from build123d import *

# Parameters (mm, degrees)
Y_KSEKLIK_EKSTR_ZYON1_DEPTH = 6
KES_EKSTR_ZYON1_DEPTH       = 28.699277969
KES_EKSTR_ZYON1_DEPTH_BACK  = 28.699277969
IZIM2_R                     = 3.5
IZIM3_R                     = 3
KES_EKSTR_ZYON2_DEPTH       = 44


with BuildPart() as part:
    # Çizim1 → Yükseklik-Ekstrüzyon1 (new body)
    with BuildSketch(Plane.XY):
        with BuildLine():
            Line((-16.5, -15), (16.5, -15))
            ThreePointArc((16.5, -15), (20.742640687, -13.242640687), (22.5, -9))
            Line((22.5, -9), (22.5, 9))
            ThreePointArc((22.5, 9), (20.742640687, 13.242640687), (16.5, 15))
            Line((16.5, 15), (-16.5, 15))
            ThreePointArc((-16.5, 15), (-20.742640687, 13.242640687), (-22.5, 9))
            Line((-22.5, 9), (-22.5, -9))
            ThreePointArc((-22.5, -9), (-20.742640687, -13.242640687), (-16.5, -15))
        make_face()
    extrude(amount=Y_KSEKLIK_EKSTR_ZYON1_DEPTH)

    # Çizim2 → Kes-Ekstrüzyon1 (cut, two sides: drawn at the far end of the back side and taken through both)
    with BuildSketch(Plane(origin=(0, 0, 0), x_dir=(0, 0, -1), z_dir=(1, 0, 0)).offset(-KES_EKSTR_ZYON1_DEPTH_BACK)):
        with Locations((-6, 10)):
            Circle(IZIM2_R)
    extrude(amount=KES_EKSTR_ZYON1_DEPTH + KES_EKSTR_ZYON1_DEPTH_BACK, mode=Mode.SUBTRACT)

    # Çizim3 → Kes-Ekstrüzyon2 (cut)
    with BuildSketch(Plane(origin=(0, 0, 0), x_dir=(-1, 0, 0), z_dir=(0, 0, -1))):
        with Locations((12.5, -5)):
            Circle(IZIM3_R)
        with Locations((-12.5, -5)):
            Circle(IZIM3_R)
    extrude(amount=-KES_EKSTR_ZYON2_DEPTH, mode=Mode.SUBTRACT)


solid = part.part
Verification items for the finished model (mm, model axes). Give positions to 0.01 mm unless a question says otherwise; leave off trailing zeros. Loops run counter-clockwise (first coordinate to the right, second up) from the corner with the lowest first, then second, coordinate; pieces in that order, holes last. Notation, with made-up numbers: (50, 31.25) - (60, 31.25) arc R10 cw to (60, 48.25) - close; hole circle Ø7 at (26, 9). An arc over 180 degrees is marked (long way). Write each question's results on one line, items separated by ' | '.
1) Sectioned sample at C-C on z = 4.75. Record the boundary of the cut face in (x, y), plus the area to 3 significant figures.
Solution:
outline: (-22.5, -9) arc R6 ccw to (-16.5, -15) - (16.5, -15) arc R6 ccw to (22.5, -9) - (22.5, 6.73) - (-22.5, 6.73) - close; (-20.72, 13.27) - (20.72, 13.27) arc R6 ccw to (16.5, 15) - (-16.5, 15) arc R6 ccw to start; hole circle Ø6 at (-12.5, -5); hole circle Ø6 at (12.5, -5) | area: 973 mm2
2) Sectioned sample at A-A on x = -12.5. Record the boundary of the cut face in (y, z), plus the area to 3 significant figures.
Solution:
outline: (-15, 0) - (-8, 0) - (-8, 6) - (-15, 6) - close; (-2, 0) - (15, 0) - (15, 6) - (13.5, 6) arc R3.5 cw to (6.5, 6) - (-2, 6) - close | area: 125 mm2
3) Material ranges on L1, parallel to Y at x = 12.5, z = 1.7; L2, parallel to Y at x = 12.5, z = 3.3; L3, parallel to Y at x = -12.5, z = 4.65, recorded low to high. Write a range as from..to.
Solution:
L1: -15..-8, -2..15 | L2: -15..-8, -2..7.77, 12.23..15 | L3: -15..-8, -2..6.77, 13.23..15
4) Sectioned sample at B-B on y = -5. Record the boundary of the cut face in (x, z).
Solution:
outline: (-22.5, 0) - (-15.5, 0) - (-15.5, 6) - (-22.5, 6) - close; (-9.5, 0) - (9.5, 0) - (9.5, 6) - (-9.5, 6) - close; (15.5, 0) - (22.5, 0) - (22.5, 6) - (15.5, 6) - close
5) Sectioned sample at D-D on z = 1.75. Record the boundary of the cut face in (x, y).
Solution:
outline: (-22.5, -9) arc R6 ccw to (-16.5, -15) - (16.5, -15) arc R6 ccw to (22.5, -9) - (22.5, 9) arc R6 ccw to (16.5, 15) - (-16.5, 15) arc R6 ccw to (-22.5, 9) - close; hole circle Ø6 at (-12.5, -5); hole circle Ø6 at (12.5, -5)
6) Mould release check, pull along X, two halves, no side actions. Record for faces 1 (the cylindrical face through (-10.29, -2.97, 2.96)), 2 (the flat face through (0, 14, 6)), 3 (the cylindrical face through (19.995, 13.877, 2.291)): pulls with the +X half, pulls with the -X half, needs draft (parallel to the pull), parting line crosses it, or undercut.
Solution:
face 1: undercut | face 2: needs draft | face 3: pulls with the +X half
